The listing builds one solid part. Answer for the finished solid, in the listing's coordinates (mm). A direction names the side the tool comes from. Round coordinates to 2 decimals unless told otherwise and drop trailing zeros. Return JSON: item names as keys, results as strings. Group by question number.
(1) Which of the six approach directions +Z, -Z, +X, -X, +Y, -Y give full straight-line access (tool end or side, diameter ignored) to faces 1 (the flat face through (2, -4.4, -118)), 2 (the flat face through (3, 1.8, 4))?
(2) Find the intervals of material crossed by line 1 along X through (y, z) = (-9.5, 240); line 2 along X through (y, z) = (-1, -60); line 3 along X through (y, z) = (-3.5, 33), in increasing order. Write a range as [from, to].
(3) Each of these flat-tipped pins is pushed along its axis until it touches: pin 1 (7 mm diameter, centred on x = 0, z = -180, fed in from -Y); pin 2 (2.5 mm diameter, centred on x = 1.5, z = 59, fed in from +Y); pin 3 (0.7 mm diameter, centred on y = 0.5, z = -37, fed in from +X). Where does it stop, or does it pass through?
(4) Determine the mould class of faces 3 (the flat face through (0, -13.9, 4)), 4 (the flat face through (0, -6, 255)), 5 (the flat face through (2, -4.4, -178)) for opening direction Z: +Z half, -Z half, draft (parallel to the pull), parting line (faces both ways), or undercut.
```python
from build123d import *

# Parameters (mm, degrees)
EXTRUDE1_DEPTH        = 255
LPATTERN1_START       = -4.39999151
LPATTERN1_OUTLINE_R   = 4
LPATTERN1_DEPTH       = 6.200000002
LPATTERN1_START_2     = -13.89999151
LPATTERN1_2_OUTLINE_R = 2.25
LPATTERN1_2_DEPTH     = 9.5


# Read off the part's stored shape, not the designer's step: LPattern1
with BuildPart() as part:
    # Sketch1 → Extrude1 (new, symmetric)
    with BuildSketch(Plane.XY):
        with BuildLine():
            Line((6.299999998, -13.89999151), (7.499999673, -12.699991836))
            Line((7.499999673, -12.699991836), (7.499999673, -10.400043863))
            Line((7.499999673, -10.400043863), (7.242437811, -10.331030371))
            ThreePointArc((7.242437811, -10.331030371), (7.108804238, -10.241739271), (7.057142573, -10.089548914))
            Line((7.057142573, -10.089548914), (7.057142573, -9.520416543))
            ThreePointArc((7.057142573, -9.520416543), (6.998907475, -9.367837553), (6.853820755, -9.292860767))
            ThreePointArc((6.853820755, -9.292860767), (5.94454945, -8.885983146), (5.43815048, -8.028146455))
            ThreePointArc((5.43815048, -8.028146455), (5.386062423, -7.939367574), (5.292449295, -7.896572271))
            ThreePointArc((5.292449295, -7.896572271), (5.190381489, -7.845596795), (5.143092926, -7.7417694))
            Line((5.143092926, -7.7417694), (4.728320242, -3.00089593))
            ThreePointArc((4.728320242, -3.00089593), (4.727832289, -2.993451213), (4.727669535, -2.985992298))
            ThreePointArc((4.727669535, -2.985992298), (4.760267524, -2.885563799), (4.845633084, -2.823424974))
            ThreePointArc((4.845633084, -2.823424974), (4.928287775, -2.764919717), (4.963356305, -2.669920448))
            ThreePointArc((4.963356305, -2.669920448), (5.395229732, -1.644926655), (6.381524191, -1.130776701))
            ThreePointArc((6.381524191, -1.130776701), (6.54675572, -1.022271679), (6.565939633, -0.825531303))
            Line((6.565939633, -0.825531303), (6.268091886, -0.007201345))
            ThreePointArc((6.268091886, -0.007201345), (6.254557346, 0.043310245), (6.249999672, 0.095404698))
            Line((6.249999672, 0.095404698), (6.249999672, 1.399956135))
            Line((6.249999672, 1.399956135), (5.850000001, 1.800008492))
            Line((5.850000001, 1.800008492), (-5.849999998, 1.800008492))
            Line((-5.849999998, 1.800008492), (-6.24999967, 1.399956135))
            Line((-6.24999967, 1.399956135), (-6.24999967, 0.095404698))
            ThreePointArc((-6.24999967, 0.095404698), (-6.254557344, 0.043310245), (-6.268091883, -0.007201345))
            Line((-6.268091883, -0.007201345), (-6.56593963, -0.825531303))
            ThreePointArc((-6.56593963, -0.825531303), (-6.546755717, -1.022271679), (-6.381524188, -1.130776701))
            ThreePointArc((-6.381524188, -1.130776701), (-5.39522973, -1.644926655), (-4.963356302, -2.669920448))
            ThreePointArc((-4.963356302, -2.669920448), (-4.928287772, -2.764919717), (-4.845633081, -2.823424974))
            ThreePointArc((-4.845633081, -2.823424974), (-4.760267522, -2.885563799), (-4.727669532, -2.985992298))
            ThreePointArc((-4.727669532, -2.985992298), (-4.727832287, -2.993451213), (-4.728320239, -3.00089593))
            Line((-4.728320239, -3.00089593), (-5.143092923, -7.7417694))
            ThreePointArc((-5.143092923, -7.7417694), (-5.190381487, -7.845596795), (-5.292449292, -7.896572271))
            ThreePointArc((-5.292449292, -7.896572271), (-5.38606242, -7.939367574), (-5.438150478, -8.028146455))
            ThreePointArc((-5.438150478, -8.028146455), (-5.944549448, -8.885983146), (-6.853820752, -9.292860767))
            ThreePointArc((-6.853820752, -9.292860767), (-6.998907472, -9.367837553), (-7.05714257, -9.520416543))
            Line((-7.05714257, -9.520416543), (-7.05714257, -10.089548914))
            ThreePointArc((-7.05714257, -10.089548914), (-7.108804235, -10.241739271), (-7.242437809, -10.331030371))
            Line((-7.242437809, -10.331030371), (-7.49999967, -10.400043863))
            Line((-7.49999967, -10.400043863), (-7.49999967, -12.699991836))
            Line((-7.49999967, -12.699991836), (-6.299999996, -13.89999151))
            Line((-6.299999996, -13.89999151), (6.299999998, -13.89999151))
        make_face()
    extrude(amount=EXTRUDE1_DEPTH, both=True)

    # Sketch2 → Hole1 (revolve, cut)
    with BuildSketch(Plane(origin=(0, 1.800008492, 240), x_dir=(0, 0, 1), z_dir=(1, 0, 0))):
        Polygon((0, 0), (0, 17.051936395), (2.25, 15.700000002), (2.25, 6.200000002), (4, 6.200000002), (4, 0), align=None)
    hole1 = revolve(axis=Axis((0, 13.110883531, 240), (0, -1, 0)), mode=Mode.SUBTRACT)

    # LPattern1 outline → LPattern1 (cut)
    with BuildSketch(Plane(origin=(0, 0, 0), x_dir=(1, 0, 0), z_dir=(0, 1, 0)).offset(LPATTERN1_START)):
        with Locations((0, -180)):
            Circle(LPATTERN1_OUTLINE_R)
        with Locations((0, -120)):
            Circle(LPATTERN1_OUTLINE_R)
        with Locations((0, -60)):
            Circle(LPATTERN1_OUTLINE_R)
        Circle(LPATTERN1_OUTLINE_R)
        with Locations((0, 60)):
            Circle(LPATTERN1_OUTLINE_R)
        with Locations((0, 120)):
            Circle(LPATTERN1_OUTLINE_R)
        with Locations((0, 180)):
            Circle(LPATTERN1_OUTLINE_R)
    extrude(amount=LPATTERN1_DEPTH, mode=Mode.SUBTRACT)

    # LPattern1 2 outline → LPattern1 2 (cut)
    with BuildSketch(Plane(origin=(0, 0, 0), x_dir=(1, 0, 0), z_dir=(0, 1, 0)).offset(LPATTERN1_START_2)):
        with Locations((0, -180)):
            Circle(LPATTERN1_2_OUTLINE_R)
        with Locations((0, -120)):
            Circle(LPATTERN1_2_OUTLINE_R)
        with Locations((0, -60)):
            Circle(LPATTERN1_2_OUTLINE_R)
        Circle(LPATTERN1_2_OUTLINE_R)
        with Locations((0, 60)):
            Circle(LPATTERN1_2_OUTLINE_R)
        with Locations((0, 120)):
            Circle(LPATTERN1_2_OUTLINE_R)
        with Locations((0, 180)):
            Circle(LPATTERN1_2_OUTLINE_R)
    extrude(amount=LPATTERN1_2_DEPTH, mode=Mode.SUBTRACT)

    # A-Mirror1: Hole1 across plane
    add(hole1.mirror(Plane.XY), mode=Mode.SUBTRACT)


solid = part.part
```
Working result:
{
 "1": {"face 1": "+Y", "face 2": "+Z, -Z, +X, -X, +Y"},
 "2": {"line 1": "x = [-7.06, -2.25], [2.25, 7.06]", "line 2": "x = [-6.56, -4], [4, 6.56]", "line 3": "x = [-4.77, 4.77]"},
 "3": {"pin 1": "stops at y = -13.9", "pin 2": "stops at y = -4.4", "pin 3": "stops at x = 6.25"},
 "4": {"face 3": "draft", "face 4": "+Z half", "face 5": "undercut"}
}
